The model under review builds one solid part; all positions refer to its coordinate system, in mm. A direction names the side the tool comes from. Coordinates: 2 decimals unless noted, no trailing zeros. Write each loop counter-clockwise with the first axis right and the second up, starting at its lowest first coordinate (ties: lowest second). Pieces come first, ordered by that corner, then holes.
```python
from build123d import *

# Parameters (mm, degrees)
SKETCH_W     = 30.8
SKETCH_H     = 10.8
PAD_DEPTH    = 1.6
SKETCH001_W  = 6
SKETCH001_H  = 6
PAD001_DEPTH = 3.5
SKETCH002_R  = 1.7
PAD002_DEPTH = 1.5


with BuildPart() as part:
    # Sketch → Pad (new body)
    with BuildSketch(Plane.XY):
        Rectangle(SKETCH_W, SKETCH_H)
    extrude(amount=-PAD_DEPTH)

    # Sketch001 → Pad001 (new body)
    with BuildSketch(Plane.XY):
        with Locations((-9, 0)):
            Rectangle(SKETCH001_W, SKETCH001_H)
        Rectangle(SKETCH001_W, SKETCH001_H)
        with Locations((9, 0)):
            Rectangle(SKETCH001_W, SKETCH001_H)
    extrude(amount=PAD001_DEPTH)

    # Sketch002 → Pad002 (new body)
    with BuildSketch(Plane.XY.offset(3.5)):
        with Locations((-9, 0)):
            Circle(SKETCH002_R)
        Circle(SKETCH002_R)
        with Locations((9, 0)):
            Circle(SKETCH002_R)
    extrude(amount=PAD002_DEPTH)


solid = part.part
```
Item 1: Take a section at B-B, the plane y = 0. Write out the cut boundary in (x, z), plus the area to 3 significant figures.
Solved:
outline: (-15.4, -1.6) - (15.4, -1.6) - (15.4, 0) - (12, 0) - (12, 3.5) - (10.7, 3.5) - (10.7, 5) - (7.3, 5) - (7.3, 3.5) - (6, 3.5) - (6, 0) - (3, 0) - (3, 3.5) - (1.7, 3.5) - (1.7, 5) - (-1.7, 5) - (-1.7, 3.5) - (-3, 3.5) - (-3, 0) - (-6, 0) - (-6, 3.5) - (-7.3, 3.5) - (-7.3, 5) - (-10.7, 5) - (-10.7, 3.5) - (-12, 3.5) - (-12, 0) - (-15.4, 0) - close
area: 128 mm2
Item 2: Take a section at D-D, the plane x = 9. Write out the cut boundary in (y, z).
Solved:
outline: (-5.4, -1.6) - (5.4, -1.6) - (5.4, 0) - (3, 0) - (3, 3.5) - (1.7, 3.5) - (1.7, 5) - (-1.7, 5) - (-1.7, 3.5) - (-3, 3.5) - (-3, 0) - (-5.4, 0) - close
Item 3: To check wall thickness, follow line 1 along X through (y, z) = (1.5, 2); line 2 along Z through (x, y) = (6.5, 4.5); line 3 along Z through (x, y) = (10.5, 2). State the ranges of each line that lie inside material, in increasing order.
Solved:
line 1: x = -12 to -6, -3 to 3, 6 to 12
line 2: z = -1.6 to 0
line 3: z = -1.6 to 3.5
Item 4: Take a section at A-A, the plane z = 1.25. Write out the cut boundary in (x, y).
Solved:
outline: (-12, -3) - (-6, -3) - (-6, 3) - (-12, 3) - close; (-3, -3) - (3, -3) - (3, 3) - (-3, 3) - close; (6, -3) - (12, -3) - (12, 3) - (6, 3) - close
Item 5: Take a section at C-C, the plane x = -6.5. Write out the cut boundary in (y, z).
Solved:
outline: (-5.4, -1.6) - (5.4, -1.6) - (5.4, 0) - (3, 0) - (3, 3.5) - (-3, 3.5) - (-3, 0) - (-5.4, 0) - close
Item 6: Mouldability with a two-part tool opening along X and no side actions: class faces 1 (the face through (-7.7, 1.4, 3.5)), 2 (the face through (9, 3, 2)), 3 (the face through (12, 0, 2)), 4 (the face through (-15.4, 0, -1)) as pulls with the +X half, pulls with the -X half, needs draft (parallel to the pull), parting line crosses it, or undercut.
Solved:
face 1: undercut
face 2: needs draft
face 3: pulls with the +X half
face 4: pulls with the -X half
Item 7: Machinability: for faces 5 (the face through (0, -3, 2)), 6 (the face through (-3, 0, 2)), 7 (the face through (10.3, 1.4, 3.5)), 8 (the face through (-9, 3, 2)), which of the approach directions +Z, -Z, +X, -X, +Y, -Y give a long, thin tool a straight path to every point of the face, cutting with its end or side? Answer none if there is none.
Solved:
face 5: +Z, +X, -X, -Y
face 6: +Z, +Y, -Y
face 7: +Z
face 8: +Z, +X, -X, +Y
Item 8: For pin 1 (1 mm diameter, centred on y = 0, z = 1.5, fed in from -X); pin 2 (3 mm diameter, centred on x = 0, z = 2, fed in from -Y); pin 3 (1 mm diameter, centred on y = 1, z = 1.5, fed in from +X), all flat-tipped, find the tip position at first contact; note any pin that passes through.
Solved:
pin 1: stops at x = -12
pin 2: stops at y = -3
pin 3: stops at x = 12
